Autodesk Inventor part; units mm, degrees
ref_plane "YZ Plane" through (0, 0, 0) normal (1, 0, 0) x (0, 1, 0)
ref_plane "XZ Plane" through (0, 0, 0) normal (0, 1, 0) x (-1, 0, 0)
ref_plane "XY Plane" through (0, 0, 0) normal (0, 0, 1) x (1, 0, 0)
sketch "Skizze" plane through (0, 0, 0) normal (1, 0, 0) x (0, 1, 0)
  circle A0 centre (0, 0) radius 1.5
  dimension "d1" = 3
extrude "Körper" add sketch "Skizze" along normal blind 10
chamfer "Fase1" distance 0.5 angle 15 1 edges at (0, -1.5, 0) measured on face at (6.6667, 1.4806, -0.2406)
chamfer "Skizze2" distance 0.5 angle 15 1 edges at (10, -1.5, 0) measured on face at (6.8333, 1.4951, -0.1207)
equation "\"d1\" = NND"
equation "\"d2\" = NLG"
equation "\"d8\" = PHH"
equation "\"d9\" = FAWI"
equation "\"d12\" = PHH"
equation "\"d4\" = PHH"
equation "\"d5\" = FAWI"
equation "\"d11\" = PHH"
equation "\"NND\" = 3"
equation "\"NLG\" = 10"
equation "\"PHH\" = 0.5"
equation "\"FAWI\" = 15deg"
equation "\"KAH\" = 0"
properties part number "ISO 2338 - 3 h8 x 10" material "Edelstahl, austenitisch"
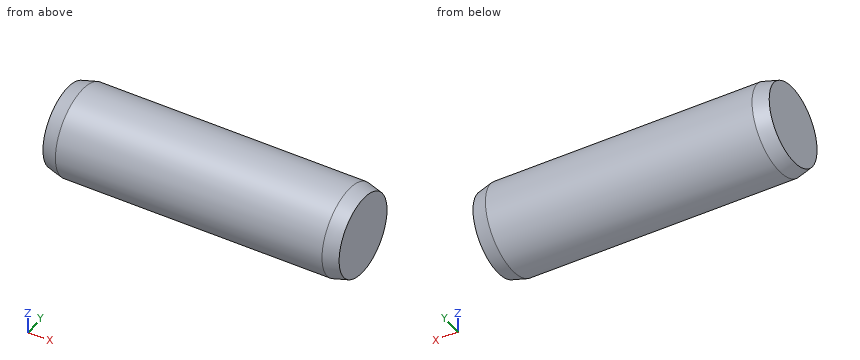
Work out the finished part from the listing and answer in its coordinate system (mm). Give positions to 0.01 mm unless a question says otherwise; leave off trailing zeros. Loops run counter-clockwise (first coordinate to the right, second up) from the corner with the lowest first, then second, coordinate; pieces in that order, holes last. Notation, with made-up numbers: M 6.25,35 L 18.25,35 A16 ccw 18.25,64 Z; hole C -24.5,37.5 d10. An arc over 180 degrees is marked long. One line per item, written item: value. Start each with the question number.
1. Find the intervals of material crossed by probe 1 along Y at (x, z) = (6.5, -1); probe 2 along Z at (x, y) = (1.5, -0.15); probe 3 along Z at (x, y) = (7, -0.5), in increasing order.
2. Find section A-A (x = 5.5). Give the vertices of the cut face in (y, z), and give its area (3 significant figures).
3. This flat-tipped pin is pushed along its axis until it touches: P1, Ø1, axis at x = 1.5, y = -1, coming from the +Z side. Where does it stop, or does it pass through?
Reported:
1. probe 1: y = -1.12 to 1.12
1. probe 2: z = -1.49 to 1.49
1. probe 3: z = -1.41 to 1.41
2. outline: C 0,0 d3
2. area: 7.07 mm²
3. P1: stops at z = 1.41
